Part model, mm, in its own coordinate system. Face numbers are marked on the shaded views. A direction names the side the tool comes from. Coordinates: 2 decimals unless noted, no trailing zeros. Loops run counter-clockwise (first coordinate to the right, second up) from the corner with the lowest first, then second, coordinate; pieces in that order, holes last. Notation, with made-up numbers: (49.5, 28) -> (93.5, 28) arc R20 cw to (93.5, 67) -> close; hole circle Ø3 at (-24, 60.5). An arc over 180 degrees is marked (long way). Use one line per item in the form item = value. Start each with the question number.
(1) Mould opens along X. For the marked faces 1, 2, 3 and 4 say: +X half, -X half, draft (parallel to the pull), parting line (faces both ways), or undercut.
(2) Band-saw the part on B-B on y = 32. Give the cut face in (x, z), then the cut area to 3 significant figures.
(3) Drill centre lines: L1, parallel to X at y = 13, z = 2.75; L2, parallel to Y at x = 30, z = 1.45; L3, parallel to Y at x = 23, z = 8. Where is each one in solid material? Low to high. Write a range as [from, to].
(4) Band-saw the part on C-C on y = 87. Give the cut face in (x, z), then the cut area to 3 significant figures.
(5) Band-saw the part on A-A on y = 57. Give the cut face in (x, z), then the cut area to 3 significant figures.
(6) Pin check, flat tips, straight feed: P1, Ø1.1, axis at x = 23.5, z = 24.5, coming from the +Y side; P2, Ø5.5, axis at x = 30, y = 57, coming from the -Z side; P3, Ø3, axis at x = 39.5, z = 7, coming from the +Y side; P4, Ø5.5, axis at x = 30, y = 29, coming from the +Z side. Stop position of each tip, or through.
(7) 3-axis set-ups, long thin cutter, end or side, ignore diameter. For the marked faces 5, 6 and 7: which of +Z, -Z, +X, -X, +Y, -Y reach the whole face in a straight line?
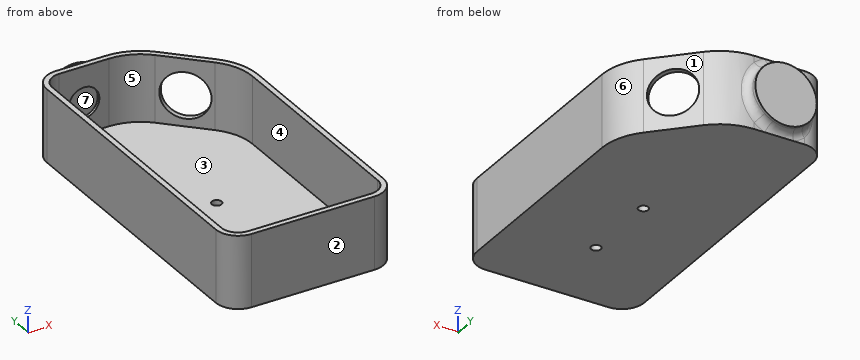
```python
from build123d import *

# Parameters (mm, degrees)
PAD_DEPTH       = 26
POCKET_DEPTH    = 24
SKETCH002_R     = 8.25
POCKET001_DEPTH = 3
SKETCH003_R     = 5.5
POCKET002_DEPTH = 3
SKETCH004_R     = 1.75
POCKET003_DEPTH = 5
SKETCH005_R     = 11
POCKET004_DEPTH = 1
SKETCH006_R     = 11
PAD001_DEPTH    = 5
FILLET_R        = 3


with BuildPart() as part:
    # Sketch → Pad (new body)
    with BuildSketch(Plane.XY):
        with BuildLine():
            Line((60, 8), (60, 82.000001))
            ThreePointArc((60, 82.000001), (58.434586, 89.869877), (53.976662, 96.541638))
            Line((40.541631, 109.976664), (53.976662, 96.541638))
            ThreePointArc((40.541631, 109.976664), (33.869872, 114.434584), (25.999999, 115.999997))
            Line((7.999999, 115.999997), (25.999999, 115.999997))
            ThreePointArc((7.999999, 115.999997), (2.343146, 113.656851), (0, 107.999998))
            Line((0, 107.999998), (0, 8))
            ThreePointArc((0, 8), (2.343146, 2.343146), (8, 0))
            Line((8, 0), (52, 0))
            ThreePointArc((52, 0), (57.656854, 2.343146), (60, 8))
        make_face()
    extrude(amount=PAD_DEPTH)

    # Sketch001 → Pocket (cut)
    with BuildSketch(Plane.XY.offset(26)):
        with BuildLine():
            ThreePointArc((8.00001, 113.999998), (3.757363, 112.242642), (2, 107.999998))
            Line((2, 107.999998), (2, 8))
            ThreePointArc((2, 8), (3.757359, 3.757359), (8, 2))
            Line((8, 2), (52, 2))
            ThreePointArc((52, 2), (56.242642, 3.757359), (58.000001, 8))
            Line((58.000001, 82), (58.000001, 8))
            ThreePointArc((58.000001, 82), (56.586824, 89.104519), (52.562435, 95.127438))
            Line((39.127419, 108.562437), (52.562435, 95.127438))
            ThreePointArc((39.127419, 108.562437), (33.104503, 112.586822), (25.99999, 113.999998))
            Line((8.00001, 113.999998), (25.99999, 113.999998))
        make_face()
    extrude(amount=-POCKET_DEPTH, mode=Mode.SUBTRACT)

    # Sketch002 → Pocket001 (cut)
    with BuildSketch(Plane(origin=(75.259141, 75.259166, 0), x_dir=(-0.707107, 0.707107, 0), z_dir=(0.707107, 0.707107, 0))):
        with Locations((39.5, 13)):
            Circle(SKETCH002_R)
    extrude(amount=-POCKET001_DEPTH, mode=Mode.SUBTRACT)

    # Sketch003 → Pocket002 (cut)
    with BuildSketch(Plane(origin=(0, 115.999997, 0), x_dir=(-1, 0, 0), z_dir=(0, 1, 0))):
        with Locations((-17, 13)):
            Circle(SKETCH003_R)
    extrude(amount=-POCKET002_DEPTH, mode=Mode.SUBTRACT)

    # Sketch004 → Pocket003 (cut)
    with BuildSketch(Plane.XY.offset(2)):
        with Locations((30, 29)):
            Circle(SKETCH004_R)
        with Locations((30, 57)):
            Circle(SKETCH004_R)
    extrude(amount=-POCKET003_DEPTH, mode=Mode.SUBTRACT)

    # Sketch005 → Pocket004 (cut)
    with BuildSketch(Plane(origin=(0, 115.999997, 0), x_dir=(-1, 0, 0), z_dir=(0, 1, 0))):
        with Locations((-17, 13)):
            Circle(SKETCH005_R)
    extrude(amount=-POCKET004_DEPTH, mode=Mode.SUBTRACT)

    # Sketch006 → Pad001 (new body)
    with BuildSketch(Plane(origin=(0, 114.999997, 0), x_dir=(-1, 0, 0), z_dir=(0, 1, 0))):
        with Locations((-17, 13)):
            Circle(SKETCH006_R)
    extrude(amount=PAD001_DEPTH)

    # Fillet
    fillet_edges = [part.edges().sort_by_distance(p)[0] for p in [
        (16.999999, 115.999997, 2),
        (28, 115.902514, 12.999999),
        (6.512058, 115.860406, 9.682926),
        (6.512058, 115.860406, 16.317074),
        (16.999999, 115.999997, 24),
    ]]
    fillet(fillet_edges, radius=FILLET_R)


solid = part.part
```
A:
q1.face_1 = +X half
q1.face_2 = draft
q1.face_3 = undercut
q1.face_4 = undercut
q2.outline = (0, 0) -> (60, 0) -> (60, 26) -> (58, 26) -> (58, 2) -> (2, 2) -> (2, 26) -> (0, 26) -> close
q2.area = 216 mm²
q3.L1 = [0, 2], [58, 60]
q3.L2 = [0, 27.25], [30.75, 55.25], [58.75, 115.61]
q3.L3 = [0, 2], [114, 120]
q4.outline = (0, 0) -> (59.38, 0) -> (59.38, 26) -> (57.31, 26) -> (57.31, 2) -> (2, 2) -> (2, 26) -> (0, 26) -> close
q4.area = 216 mm²
q5.outline = (0, 0) -> (28.25, 0) -> (28.25, 2) -> (2, 2) -> (2, 26) -> (0, 26) -> close; (31.75, 0) -> (60, 0) -> (60, 26) -> (58, 26) -> (58, 2) -> (31.75, 2) -> close
q5.area = 209 mm²
q6.P1 = 116.32
q6.P2 = 0
q6.P3 = 112.14
q6.P4 = 2
q7.face_5 = +Z
q7.face_6 = +Z, -Z, +X, +Y
q7.face_7 = none
